Verification items for the finished model (mm, model axes). A direction names the side the tool comes from. Coordinates: 2 decimals unless noted, no trailing zeros. Write each loop counter-clockwise with the first axis right and the second up, starting at its lowest first coordinate (ties: lowest second). Pieces come first, ordered by that corner, then holes.
```python
from build123d import *

# Parameters (mm, degrees)
F0_R     = 4
F0_R_2   = 2.6
F1_DEPTH = 15
F2_START = 6
F0_W     = 4.4
F0_H     = 2.5
F2_DEPTH = 9
F3_START = 6
F3_DEPTH = 6


# Not quite as in the source:
# - a fillet or chamfer that OpenCascade refuses, or shapes differently, is made with other operations: its cross-section is extruded or revolved along the edge and cut away or added


with BuildPart() as f1:
    # F0 (on Top) → F1 (new body)
    with BuildSketch(Plane.XY):
        Circle(F0_R)
        Circle(F0_R_2, mode=Mode.SUBTRACT)
    extrude(amount=F1_DEPTH)

    # F0 (on Top) → F2 (join)
    with BuildSketch(Plane.XY.offset(F2_START)):
        Circle(F0_R_2)
        Rectangle(F0_W, F0_H, mode=Mode.SUBTRACT)
    extrude(amount=F2_DEPTH)

    # F0 (on Top) → F3 (join)
    with BuildSketch(Plane.XY.offset(F3_START)):
        Rectangle(F0_W, F0_H)
    extrude(amount=F3_DEPTH)

    # F4: chamfer of 1.5 on 1 edges, made by hand

    # F4_s1 → F4_t2 (revolve, cut)
    with BuildSketch(Plane.XZ):
        Polygon((4, 13.5), (2.5, 15), (4, 15), align=None)
    revolve(axis=Axis((0, 0, 15), (0, 0, 1)), mode=Mode.SUBTRACT)


solid = f1.part
```
1. Gauge pin test, flat ends, axial feed: P1, Ø2.5, axis at x = -0.5, z = 14, coming from the -Y side; P2, Ø1.6, axis at x = 0, y = 0.5, coming from the -Z side; P3, Ø0.8, axis at x = -0.5, y = 0.5, coming from the +Z side; P4, Ø1, axis at y = -2, z = 8.5, coming from the +X side. Record the tip position at first contact, or that the pin passes through.
2. Sectioned sample at B-B, the plane z = 1.5. Record the boundary of the cut face in (x, y), and give its area (3 significant figures).
3. Draft check along X on faces 1 (the flat face through (0, -2, 15)), 2 (the flat face through (2.2, 0, 13)), 3 (the cylindrical face through (-0.867, -3.905, 6.656)). Enter one of: pulls with the +X half, pulls with the -X half, needs draft (parallel to the pull), parting line crosses it, or undercut.
4. Sectioned sample at A-A, the plane x = 0. Record the boundary of the cut face in (y, z).
5. Material ranges on L1, parallel to Y at x = 0, z = 4.8; L2, parallel to Z at x = 1.5, y = 1; L3, parallel to X at y = -0.75, z = 5, recorded low to high.
6. Sectioned sample at D-D, the plane z = 7. Record the boundary of the cut face in (x, y), and give its area (3 significant figures).
7. Sectioned sample at C-C, the plane y = 0. Record the boundary of the cut face in (x, z), and give its area (4 significant figures).
8. Tool access check on faces 4 (the flat face through (-2.2, 0, 13)), 5 (the flat face through (3, 0, 0)), 6 (the cylindrical face through (-0.338, 2.578, 2.958)). Record the directions out of +Z, -Z, +X, -X, +Y, -Y that give a thin tool (end or side, any length) a straight path to the whole face; none if there is none.
Outcome:
1. P1: stops at y = -4
1. P2: stops at z = 6
1. P3: stops at z = 12
1. P4: stops at x = 3.71
2. outline: circle Ø8 at (0, 0); hole circle Ø5.2 at (0, 0)
2. area: 29.0 mm2
3. face 1: needs draft
3. face 2: undercut
3. face 3: parting line crosses it
4. outline: (-4, 0) - (-2.6, 0) - (-2.6, 6) - (2.6, 6) - (2.6, 0) - (4, 0) - (4, 13.5) - (2.5, 15) - (1.25, 15) - (1.25, 12) - (-1.25, 12) - (-1.25, 15) - (-2.5, 15) - (-4, 13.5) - close
5. L1: y = -4 to -2.6, 2.6 to 4
5. L2: z = 6 to 12
5. L3: x = -3.93 to -2.49, 2.49 to 3.93
6. outline: circle Ø8 at (0, 0)
6. area: 50.3 mm2
7. outline: (-4, 0) - (-2.6, 0) - (-2.6, 6) - (2.6, 6) - (2.6, 0) - (4, 0) - (4, 13.5) - (2.5, 15) - (2.2, 15) - (2.2, 12) - (-2.2, 12) - (-2.2, 15) - (-2.5, 15) - (-4, 13.5) - close
7. area: 73.35 mm2
8. face 4: +Z
8. face 5: -Z, +X, -X, +Y, -Y
8. face 6: -Z
